Build history of the part. All positions in model axes, mm. A direction names the side the tool comes from. Round coordinates to 2 decimals unless told otherwise and drop trailing zeros. Write each loop counter-clockwise with the first axis right and the second up, starting at its lowest first coordinate (ties: lowest second). Pieces come first, ordered by that corner, then holes. Notation, with made-up numbers: (5.25, -17) -> (59.25, -17) arc R21 cw to (59.25, 21) -> close; hole circle Ø9 at (2, 66.25). An arc over 180 degrees is marked (long way). Answer in a Markdown table with one row per item.
Autodesk Inventor part; units mm, degrees
ref_plane "YZ Plane" through (0, 0, 0) normal (1, 0, 0) x (0, 1, 0)
ref_plane "XZ Plane" through (0, 0, 0) normal (0, 1, 0) x (-1, 0, 0)
ref_plane "XY Plane" through (0, 0, 0) normal (0, 0, 1) x (1, 0, 0)
sketch "Sketch1" plane through (0, 0, 0) normal (0, 1, 0) x (-1, 0, 0)
  line L0 (0, 0) -> (144.25, 0)
  line L1 (144.25, 0) -> (144.25, -204.25)
  line L2 (144.25, -204.25) -> (0, -204.25)
  line L3 (0, -204.25) -> (0, 0)
  line L4 (132.25, -12) -> (12, -12) construction
  line L5 (12, -12) -> (12, -192.25) construction
  line L6 (12, -192.25) -> (132.25, -192.25) construction
  line L7 (132.25, -192.25) -> (132.25, -12) construction
  circle A0 centre (135.25, -27) radius 3 construction
  circle A1 centre (122.25, -9) radius 3 construction
  circle A2 centre (122.25, -9) radius 2.925
  circle A3 centre (135.25, -27) radius 2.925
  circle A4 centre (135.25, -177.25) radius 3 construction
  circle A5 centre (122.25, -195.25) radius 3 construction
  circle A6 centre (22, -195.25) radius 3 construction
  circle A7 centre (9, -177.25) radius 3 construction
  circle A8 centre (22, -195.25) radius 2.925
  circle A9 centre (9, -177.25) radius 2.925
  circle A10 centre (135.25, -177.25) radius 2.925
  circle A11 centre (122.25, -195.25) radius 2.925
  circle A12 centre (22, -9) radius 3 construction
  circle A13 centre (9, -27) radius 3 construction
  circle A14 centre (22, -9) radius 2.925
  circle A15 centre (9, -27) radius 2.925
  point P0 (144.25, -102.125)
  point P1 (132.25, -102.125)
  point P2 (72.125, -12)
  point P3 (72.125, 0)
  dimension "width" = 204.25
  dimension "height" = 144.25
  dimension "stencilW" = 180.25
  dimension "stencilH" = 120.25
  dimension "d14" = 6
  dimension "d15" = 6
  dimension "kerf" = 0.075
  dimension "d17" = 0.075
  dimension "cornerW" = 15
  dimension "cornerH" = 10
  dimension "d20" = 6
  dimension "d21" = 6
  dimension "d22" = 6
  dimension "d23" = 6
  dimension "d24" = 10
  dimension "d25" = 15
  dimension "d26" = 10
  dimension "d27" = 15
  dimension "d28" = 0.075
  dimension "d29" = 0.075
  dimension "d30" = 0.075
  dimension "d31" = 0.075
  dimension "d32" = 6
  dimension "d33" = 6
  dimension "d34" = 15
  dimension "d35" = 10
  dimension "d36" = 0.075
  dimension "d37" = 0.075
extrude "Extrusion1" add sketch "Sketch1" along normal blind 3
fillet "Fillet1" radius 6 4 edges at (0, 1.5, 0) (-144.25, 1.5, 0) (0, 1.5, -204.25) (-144.25, 1.5, -204.25)
sketch "Sketch2" plane through (0, 3, 0) normal (0, 1, 0) x (1, 0, 0)
  line L0 (-72.125, -7.125) -> (-72.125, 7.125) construction
  line L1 (-6, 0) -> (-138.25, 0)
  line L2 (-59.625, -7.125) -> (-59.625, 7.125)
  line L3 (-84.625, 7.125) -> (-84.625, -7.125)
  arc A0 (-84.625, -7.125) -> (-59.625, -7.125) centre (-72.125, -7.125) ccw
  arc A1 (-59.625, 7.125) -> (-84.625, 7.125) centre (-72.125, 7.125) ccw
  line L4 (-72.125, 0) -> (-57.875, 0) construction
  line L5 (-144.25, 198.25) -> (-144.25, 6) construction
  line L6 (-144.25, 102.125) -> (0, 102.125) construction
  line L7 (0, 6) -> (0, 198.25) construction
  line L8 (-72.125, 211.375) -> (-72.125, 197.125) construction
  line L9 (-59.625, 211.375) -> (-59.625, 197.125)
  line L10 (-84.625, 197.125) -> (-84.625, 211.375)
  arc A2 (-59.625, 211.375) -> (-84.625, 211.375) centre (-72.125, 211.375) ccw
  arc A3 (-84.625, 197.125) -> (-59.625, 197.125) centre (-72.125, 197.125) ccw
  line L11 (-100.1727, 19.625) -> (-55, 19.625) construction
  line L12 (-92.5099, 184.625) -> (-51.3219, 184.625) construction
  point P0 (0, 0)
  dimension "d42" = 90
  dimension "fingerW" = 25
  dimension "d47" = 165
extrude "Extrusion2" cut sketch "Sketch2" against normal blind 3
fillet "Fillet2" radius 6 4 edges at (-84.625, 1.5, 0) (-59.625, 1.5, 0) (-84.625, 1.5, -204.25) (-59.625, 1.5, -204.25)
sketch "Sketch3" plane through (0, 3, 0) normal (0, 1, 0) x (1, 0, 0)
  arc A0 (-59.625, 7.125) -> (-84.625, 7.125) centre (-72.125, 7.125) ccw construction
  arc A1 (-84.625, 197.125) -> (-59.625, 197.125) centre (-72.125, 197.125) ccw construction
  line L0 (-144.25, 198.25) -> (-144.25, 6) construction
  line L1 (0, 6) -> (0, 198.25) construction
  arc A2 (-59.625, 7.125) -> (-84.625, 7.125) centre (-72.125, 7.125) ccw construction
  line L2 (-72.125, 19.625) -> (-72.125, 184.625)
  line L3 (-144.25, 102.125) -> (0, 102.125)
  point P0 (0, 0)
sketch "Sketch4" plane through (0, 3, 0) normal (0, 1, 0) x (1, 0, 0)
  circle A0 centre (-135.25, 77.0833) radius 2
  circle A1 centre (-135.25, 127.1667) radius 2
  arc A2 (-53.625, 204.25) -> (-59.625, 198.25) centre (-53.625, 198.25) ccw construction
  line L0 (-59.625, 198.25) -> (-59.625, 197.125) construction
  arc A3 (-84.625, 197.125) -> (-59.625, 197.125) centre (-72.125, 197.125) ccw construction
  line L1 (-84.625, 197.125) -> (-84.625, 198.25) construction
  arc A4 (-84.625, 198.25) -> (-90.625, 204.25) centre (-90.625, 198.25) ccw construction
  line L2 (-90.625, 204.25) -> (-138.25, 204.25) construction
  arc A5 (-138.25, 204.25) -> (-144.25, 198.25) centre (-138.25, 198.25) ccw construction
  line L3 (-144.25, 198.25) -> (-144.25, 6) construction
  arc A6 (-144.25, 6) -> (-138.25, 0) centre (-138.25, 6) ccw construction
  line L4 (-138.25, 0) -> (-90.625, 0) construction
  arc A7 (-90.625, 0) -> (-84.625, 6) centre (-90.625, 6) ccw construction
  line L5 (-84.625, 6) -> (-84.625, 7.125) construction
  arc A8 (-59.625, 7.125) -> (-84.625, 7.125) centre (-72.125, 7.125) ccw construction
  line L6 (-59.625, 7.125) -> (-59.625, 6) construction
  arc A9 (-59.625, 6) -> (-53.625, 0) centre (-53.625, 6) ccw construction
  line L7 (-53.625, 0) -> (-6, 0) construction
  arc A10 (-6, 0) -> (0, 6) centre (-6, 6) ccw construction
  line L8 (0, 6) -> (0, 198.25) construction
  arc A11 (0, 198.25) -> (-6, 204.25) centre (-6, 198.25) ccw construction
  line L9 (-6, 204.25) -> (-53.625, 204.25) construction
  circle A12 centre (-9, 27) radius 2.925 construction
  circle A13 centre (-22, 9) radius 2.925 construction
  circle A14 centre (-122.25, 195.25) radius 2.925 construction
  circle A15 centre (-135.25, 177.25) radius 2.925 construction
  circle A16 centre (-9, 177.25) radius 2.925 construction
  circle A17 centre (-22, 195.25) radius 2.925 construction
  circle A18 centre (-135.25, 27) radius 2.925 construction
  circle A19 centre (-122.25, 9) radius 2.925 construction
  circle A20 centre (-9, 77.0833) radius 2
  circle A21 centre (-9, 127.1667) radius 2
  circle A22 centre (-97.125, 9) radius 2
  circle A23 centre (-47.125, 9) radius 2
  circle A24 centre (-47.125, 195.25) radius 2
  circle A25 centre (-97.125, 195.25) radius 2
  point P0 (0, 0)
  dimension "d48" = 4
  dimension "d49" = 4
  dimension "d50" = 50.0833
  dimension "d51" = 50.0833
  dimension "d52" = 50.0833
  dimension "d53" = 4
  dimension "d54" = 4
  dimension "d55" = 4
  dimension "d56" = 4
  dimension "d57" = 4
  dimension "d58" = 4
  dimension "d59" = 50
  dimension "d60" = 25.125
  dimension "d61" = 25.125
extrude "Extrusion3" cut sketch "Sketch4" against normal blind 3
equation "\"width\" = stencilW + 4 * pinD"
equation "\"height\" = stencilH + 4 * pinD"
equation "\"d14\" = pinD"
equation "\"d15\" = pinD"
equation "\"d17\" = kerf"
equation "\"d20\" = pinD"
equation "\"d21\" = pinD"
equation "\"d22\" = pinD"
equation "\"d23\" = pinD"
equation "\"d24\" = cornerH"
equation "\"d25\" = cornerW"
equation "\"d26\" = cornerH"
equation "\"d27\" = cornerW"
equation "\"d28\" = kerf"
equation "\"d29\" = kerf"
equation "\"d30\" = kerf"
equation "\"d31\" = kerf"
equation "\"d32\" = pinD"
equation "\"d33\" = pinD"
equation "\"d34\" = cornerW"
equation "\"d35\" = cornerH"
equation "\"d36\" = kerf"
equation "\"d37\" = kerf"
equation "\"d40\" = pinD"
equation "\"d46\" = pinD"
equation "\"d50\" = d52"
equation "\"d51\" = d50"
equation "\"d60\" = d61"
properties part number "base"
Q1. Saw through at B-B on x = -122.25. Write the cut outline in (y, z) (3 decimals), plus the area to 3 significant figures.
A:
| item | result |
|---|---|
| outline | (0, -204.25) -> (3, -204.25) -> (3, -198.175) -> (0, -198.175) -> close; (0, -192.325) -> (3, -192.325) -> (3, -11.925) -> (0, -11.925) -> close; (0, -6.075) -> (3, -6.075) -> (3, 0) -> (0, 0) -> close |
| area | 578 mm² |
Q2. Which spindle directions (+Z, -Z, +X, -X, +Y, -Y) get a long thin tool onto all of the face, cutting with end or side? Do faces 4 (the cylindrical face through (-132.328, 1.479, -27.129)), 5 (the cylindrical face through (-57.91, 1.52, -1.8)), 6 (the cylindrical face through (-57.82, 1.52, -202.54)). Say none if no direction does.
A:
| item | result |
|---|---|
| face 4 | +Y, -Y |
| face 5 | +Z, +Y, -Y |
| face 6 | -Z, +Y, -Y |
Q3. Saw through at C-C on z = -15.5. Write the cut outline in (x, y).
A:
| item | result |
|---|---|
| outline | (-144.25, 0) -> (-81.4, 0) -> (-81.4, 3) -> (-144.25, 3) -> close; (-62.85, 0) -> (0, 0) -> (0, 3) -> (-62.85, 3) -> close |
Q4. Saw through at A-A on z = -177.25. Write the cut outline in (x, y) (3 decimals), plus the area to 3 significant figures.
A:
| item | result |
|---|---|
| outline | (-144.25, 0) -> (-138.175, 0) -> (-138.175, 3) -> (-144.25, 3) -> close; (-132.325, 0) -> (-11.925, 0) -> (-11.925, 3) -> (-132.325, 3) -> close; (-6.075, 0) -> (0, 0) -> (0, 3) -> (-6.075, 3) -> close |
| area | 398 mm² |
Q5. Two-plate mould, pull along X, no slides. Class faces 1 (the flat face through (-71, 0, -101)), 2 (the cylindrical face through (-1.804, 1.521, -1.711)), 3 (the cylindrical face through (-96.202, 1.521, -193.476)): released by +X, released by -X, zero draft, split by the parting line, or undercut.
A:
| item | result |
|---|---|
| face 1 | zero draft |
| face 2 | released by +X |
| face 3 | undercut |
Q6. Wall check: line 1 (Z direction, x = -22, y = 2.1) (3 decimals); line 2 (Z direction, x = -135.25, y = 2.2) (3 decimals); line 3 (X direction, y = 1.7, z = -195.25) (3 decimals). Give the ranges that are in metal, low to high. Write a range as [from, to].
A:
| item | result |
|---|---|
| line 1 | [-204.25, -198.175], [-192.325, -11.925], [-6.075, 0] |
| line 2 | [-204.25, -180.175], [-174.325, -129.167], [-125.167, -79.083], [-75.083, -29.925], [-24.075, 0] |
| line 3 | [-144.25, -125.175], [-119.325, -99.125], [-95.125, -84.484], [-59.766, -49.125], [-45.125, -24.925], [-19.075, 0] |
Q7. Saw through at D-D on y = 1. State how many separate pieces and enclosed holes the cut face has, plus the area to 3 significant figures.
A:
| item | result |
|---|---|
| separate pieces | 1 |
| enclosed holes | 16 |
| area | 28,200 mm² |
Q8. Drop flat-ended pins along their axis: P1, Ø5, axis at x = -9, z = -77.08, coming from the -Y side; P2, Ø1.5, axis at x = -56, y = 2, coming from the +Z side. Give the stop position or say it passes through.
A:
| item | result |
|---|---|
| P1 | y = 0 |
| P2 | z = -0.22 |
